The drawing under review shows one solid part. Ordinate dimensions are in mm from its lowest x, y, z. A direction names the side the tool comes from. Coordinates: 2 decimals unless noted, no trailing zeros. Write each loop counter-clockwise with the first axis right and the second up, starting at its lowest first coordinate (ties: lowest second). Pieces come first, ordered by that corner, then holes. Notation, with made-up numbers: (12, 43) -> (52, 43) arc R28 cw to (52, 76) -> close; hole circle Ø9 at (-37.5, 43). An arc over 180 degrees is marked (long way). One line per item, written item: value. Start each with the question number.
1) Add section A-A (x = 31.5). State the section outline as (y, z) points (3 decimals), and give its area (3 significant figures).
2) For pin 1 Ø2.5 at (x, y) = (18.5, 5) entering from -Z; pin 2 Ø1.4 at (y, z) = (21, 3.5) entering from -X; pin 3 Ø1.5 at (y, z) = (18.5, 3.5) entering from -X; pin 4 Ø1 at (x, z) = (23.5, 1) entering from -Y, all flat-tipped, find the tip position at first contact; note any pin that passes through.
3) Mouldability with a two-part tool opening along Y and no side actions: class the marked faces 6, 7 and 8 as released by +Y, released by -Y, zero draft, split by the parting line, or undercut.
4) Machinability: for the marked faces 1, 2, 3, 4 and 5, which of the approach directions +Z, -Z, +X, -X, +Y, -Y give a long, thin tool a straight path to every point of the face, cutting with its end or side? Answer none if there is none.
5) Add section B-B (x = 18.5). State the section outline as (y, z) points (3 decimals), and give its area (4 significant figures).
6) For probe 1 along Y at (x, z) = (18.5, 1.25) (3 decimals); probe 2 along Y at (x, z) = (4, 0.35); probe 3 along X at (y, z) = (35, 1.2), list the stretches that pass through material, from the lowest coordinate up. Write a range as from..to.
7) Add section D-D (z = 1.1). State how many separate pieces and enclosed holes the cut face has, and give its area (3 significant figures).
8) Add section C-C (y = 33.5). State the section outline as (x, z) points.
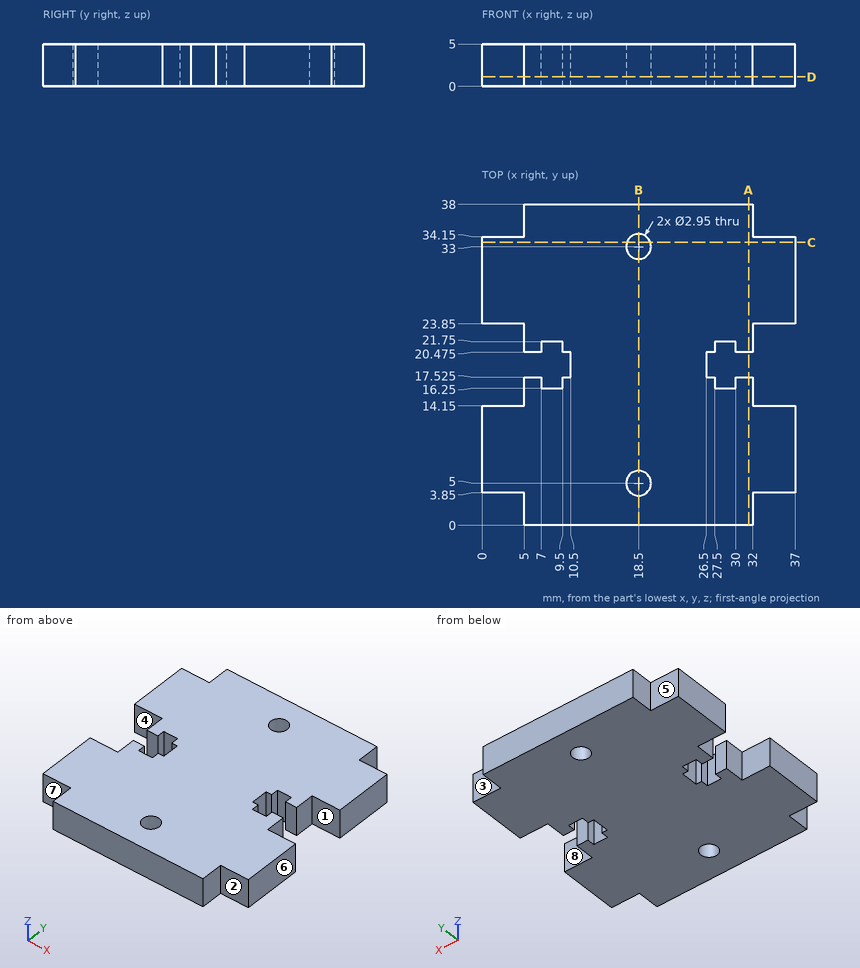
Numbers:
1. outline: (0, 0) -> (17.525, 0) -> (17.525, 5) -> (0, 5) -> close; (20.475, 0) -> (38, 0) -> (38, 5) -> (20.475, 5) -> close
1. area: 175 mm²
2. pin 1: through
2. pin 2: x = 5
2. pin 3: x = 10.5
2. pin 4: y = 0
3. face 6: zero draft
3. face 7: released by -Y
3. face 8: undercut
4. face 1: +Z, -Z, +X
4. face 2: +Z, -Z, +X, -Y
4. face 3: +Z, -Z, +X, +Y
4. face 4: +Z, -Z, -X
4. face 5: +Z, -Z, -X, +Y
5. outline: (0, 0) -> (3.525, 0) -> (3.525, 5) -> (0, 5) -> close; (6.475, 0) -> (31.525, 0) -> (31.525, 5) -> (6.475, 5) -> close; (34.475, 0) -> (38, 0) -> (38, 5) -> (34.475, 5) -> close
5. area: 160.5 mm²
6. probe 1: 0..3.525, 6.475..31.525, 34.475..38
6. probe 2: 3.85..14.15, 23.85..34.15
6. probe 3: 5..32
7. separate pieces: 1
7. enclosed holes: 2
7. area: 1,170 mm²
8. outline: (0, 0) -> (17.11, 0) -> (17.11, 5) -> (0, 5) -> close; (19.89, 0) -> (37, 0) -> (37, 5) -> (19.89, 5) -> close
